```python
from build123d import *

# Parameters (mm, degrees)
F0_W      = 60
F0_H      = 180
F0_R      = 12.75
F0_R_2    = 2.5
F1_DEPTH  = 3
F2_R      = 18
F2_R_2    = 12.75
F3_DEPTH  = 2.6
F4_W      = 60
F4_H      = 70
F4_W_2    = 54
F4_H_2    = 64
F5_DEPTH  = 40
F6_W      = 5
F6_H      = 5
F6_W_2    = 10
F6_H_2    = 3
F6_W_3    = 3
F6_H_3    = 10
F7_DEPTH  = 37
F8_R      = 1.6
F9_DEPTH  = 28
F10_W     = 3
F10_H     = 70
F11_DEPTH = 70
F13_R     = 20.5
F14_DEPTH = 3
F16_DEPTH = 5
F17_R     = 3.075
F18_DEPTH = 6
F19_R     = 3.1
F20_DEPTH = 6
F22_DEPTH = 5


with BuildPart() as f1:
    # F0 (on Front) → F1 (new body)
    with BuildSketch(Plane.XZ):
        Rectangle(F0_W, F0_H)
        with Locations((0, -55)):
            Circle(F0_R, mode=Mode.SUBTRACT)
        with Locations((-17.5, 30)):
            Circle(F0_R_2, mode=Mode.SUBTRACT)
        with Locations((-17.5, 75)):
            Circle(F0_R_2, mode=Mode.SUBTRACT)
        with Locations((17.5, 30)):
            Circle(F0_R_2, mode=Mode.SUBTRACT)
        with Locations((17.5, 75)):
            Circle(F0_R_2, mode=Mode.SUBTRACT)
    extrude(amount=-F1_DEPTH)

    # F2 (on face) → F3 (join)
    with BuildSketch(Plane.XZ):
        with Locations((0, -55)):
            Circle(F2_R)
        with Locations((0, -55)):
            Circle(F2_R_2, mode=Mode.SUBTRACT)
    extrude(amount=F3_DEPTH)

    # F4 (on face) → F5 (join)
    with BuildSketch(Plane.XZ):
        with Locations((0, -55)):
            Rectangle(F4_W, F4_H)
        with Locations((0, -55)):
            Rectangle(F4_W_2, F4_H_2, mode=Mode.SUBTRACT)
    extrude(amount=F5_DEPTH)

    # F6 (on face) → F7 (join)
    with BuildSketch(Plane.XZ):
        with Locations((-24.5, -25.5)):
            Rectangle(F6_W, F6_H)
        with Locations((0, -24.5)):
            Rectangle(F6_W_2, F6_H_2)
        with Locations((24.5, -25.5)):
            Rectangle(F6_W, F6_H)
        with Locations((25.5, -55)):
            Rectangle(F6_W_3, F6_H_3)
        with Locations((-25.5, -55)):
            Rectangle(F6_W_3, F6_H_3)
        with Locations((24.5, -84.5)):
            Rectangle(F6_W, F6_H)
        with Locations((0, -85.5)):
            Rectangle(F6_W_2, F6_H_2)
        with Locations((-24.5, -84.5)):
            Rectangle(F6_W, F6_H)
    extrude(amount=F7_DEPTH)

    # F8 (on face) → F9 (cut)
    with BuildSketch(Plane.XZ.offset(37)):
        with Locations((24.5, -25.5)):
            Circle(F8_R)
        with Locations((-24.5, -25.5)):
            Circle(F8_R)
        with Locations((24.5, -84.5)):
            Circle(F8_R)
        with Locations((-24.5, -84.5)):
            Circle(F8_R)
    extrude(amount=-F9_DEPTH, mode=Mode.SUBTRACT)

    # F10 (on face) → F11 (join)
    with BuildSketch(Plane.YZ.offset(30)):
        with Locations((1.5, -55)):
            Rectangle(F10_W, F10_H)
    extrude(amount=F11_DEPTH)

    # F13 (on face) → F14 (cut, through all)
    with BuildSketch(Plane.XZ):
        with Locations((65, -55)):
            Circle(F13_R)
    extrude(amount=-F14_DEPTH, mode=Mode.SUBTRACT)

    # F15 (on face) → F16 (join)
    with BuildSketch(Plane.XZ):
        Polygon((100, -20), (30, -20), (30, -23), (97, -23), (97, -87), (30, -87), (30, -90), (100, -90), (100, -87), (100, -23), align=None)
    extrude(amount=F16_DEPTH)

    # F17 (on face) → F18 (cut, through all)
    with BuildSketch(Plane.YZ.offset(30)):
        with Locations((-22.5, -55)):
            Circle(F17_R)
    extrude(amount=-F18_DEPTH, mode=Mode.SUBTRACT)

    # F19 (on face) → F20 (cut, through all)
    with BuildSketch(Plane.XY.offset(-20)):
        with Locations((0, -20)):
            Circle(F19_R)
    extrude(amount=-F20_DEPTH, mode=Mode.SUBTRACT)

    # F21 (on face) → F22 (join)
    with BuildSketch(Plane.XZ):
        Polygon((30, -20), (30, 90), (27, 90), (21.684641, 90), (-27, 90), (-30, 90), (-30, -20), (-27, -20), (-27, 87), (27, 87), (27, -20), align=None)
    extrude(amount=F22_DEPTH)


solid = f1.part
```
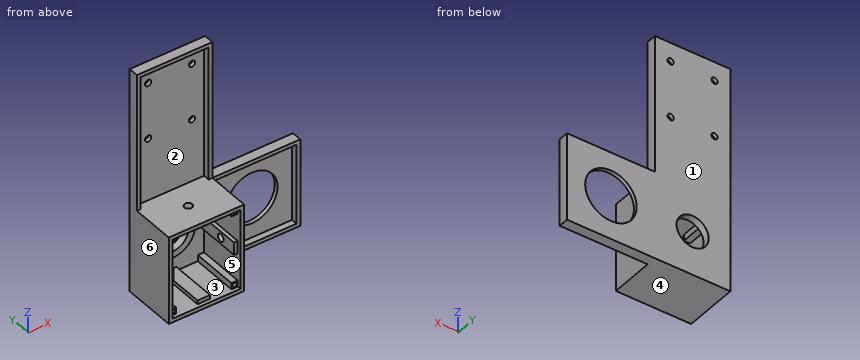
Work out the finished part from the listing and answer in its coordinate system (mm). Face numbers are marked on the shaded views. A direction names the side the tool comes from. Give positions to 0.01 mm unless a question says otherwise; leave off trailing zeros. Loops run counter-clockwise (first coordinate to the right, second up) from the corner with the lowest first, then second, coordinate; pieces in that order, holes last. Notation, with made-up numbers: (70.25, 87.5) -> (97.25, 87.5) arc R15 cw to (97.25, 92.5) -> close; hole circle Ø6 at (-37.5, 59). An arc over 180 degrees is marked (long way). Write item = value, one per line. Start each with the question number.
(1) Find section B-B on x = 0. Give the vertices of the cut face in (y, z), and give its area (3 significant figures).
(2) Which of the six approach directions +Z, -Z, +X, -X, +Y, -Y give full straight-line access (tool end or side, diameter ignored) to the marked faces 1 and 2?
(3) Find section C-C on z = -10. Give the vertices of the cut face in (x, y).
(4) The mould has two halves that part along Z. Classify the marked faces 3, 4, 5 and 6: +Z half, -Z half, draft (parallel to the pull), parting line (faces both ways), or undercut.
(5) Given pin 1 Ø1.5 at (y, z) = (-15, -24.5) entering from +X; pin 2 Ø3.5 at (x, z) = (24.5, -25) entering from -Y; pin 3 Ø1.6 at (x, z) = (24.5, -84.5) entering from -Y, each flat-ended and moving along its own axis, determine where each tip first touches the part or whether it passes through.
(6) Find section D-D on x = 39.5. Give the vertices of the cut face in (y, z).
(7) Find section A-A on z = -55. Give the number of separate pieces and of enclosed holes in the cut face, and give its area (3 significant figures).
(8) Find the intervals of material crossed by probe 1 along Z at (x, y) = (24.5, -30.75); probe 2 along X at (y, z) = (-19.5, -84.5); probe 3 along Z at (x, y) = (-17.5, 1.85), in increasing order. Write a range as from..to.
From the geometry:
q1.outline = (-40, -90) -> (3, -90) -> (3, -67.75) -> (-2.6, -67.75) -> (-2.6, -73) -> (0, -73) -> (0, -84) -> (-37, -84) -> (-37, -87) -> (-40, -87) -> close; (-40, -23) -> (-37, -23) -> (-37, -26) -> (-23.1, -26) -> (-23.1, -20) -> (-40, -20) -> close; (-16.9, -26) -> (0, -26) -> (0, -37) -> (-2.6, -37) -> (-2.6, -42.25) -> (3, -42.25) -> (3, 90) -> (-5, 90) -> (-5, 87) -> (0, 87) -> (0, -20) -> (-16.9, -20) -> close
q1.area = 931 mm^2
q2.face_1 = +Z, -Z, +X, -X, +Y
q2.face_2 = -Y
q3.outline = (-30, -5) -> (-27, -5) -> (-27, 0) -> (27, 0) -> (27, -5) -> (30, -5) -> (30, 3) -> (-30, 3) -> close
q4.face_3 = undercut
q4.face_4 = -Z half
q4.face_5 = undercut
q4.face_6 = draft
q5.pin_1 = 30
q5.pin_2 = -37
q5.pin_3 = -9
q6.outline = (-5, -90) -> (3, -90) -> (3, -20) -> (-5, -20) -> (-5, -23) -> (0, -23) -> (0, -87) -> (-5, -87) -> close
q7.separate_pieces = 4
q7.enclosed_holes = 0
q7.area = 658 mm^2
q8.probe_1 = -90..-86.1, -82.9..-82, -60..-50, -28..-27.1, -23.9..-20
q8.probe_2 = -30..-26.1, -22.9..-22, -5..5, 22..22.9, 26.1..30
q8.probe_3 = -90..27.5, 32.5..72.5, 77.5..90
